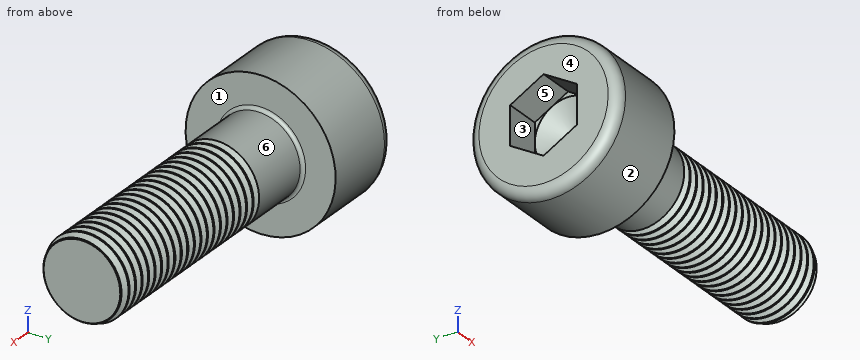
from build123d import *

# Parameters (mm, degrees)
SKETCH1_R           = 2.25
BASEHEAD_DEPTH      = 2.5
SKETCH2_R           = 1.25
BASEBODY_DEPTH      = 8
HEXAGONSOCKET_DEPTH = 1.1
HEADFILLET_R        = 0.1
TOPFILLET_R         = 0.3125
CHAMFER1_SIZE       = 0.1
LPATTERN10_COUNT    = 21
LPATTERN10_PITCH    = 0.2922


with BuildPart() as part:
    # Sketch1 → BaseHead (new body)
    with BuildSketch(Plane(origin=(0, 0, 0), x_dir=(0, 0, -1), z_dir=(1, 0, 0))):
        Circle(SKETCH1_R)
    extrude(amount=BASEHEAD_DEPTH)

    # Sketch2 → BaseBody (add)
    with BuildSketch(Plane(origin=(2.5, 0, 0), x_dir=(0, 0, -1), z_dir=(1, 0, 0))):
        Circle(SKETCH2_R)
    extrude(amount=BASEBODY_DEPTH)

    # Sketch3 → HexagonSocket (cut)
    with BuildSketch(Plane(origin=(0, 0, 0), x_dir=(0, 0, -1), z_dir=(1, 0, 0))):
        Polygon((1.154700538, 0), (0.577350269, 1), (-0.577350269, 1), (-1.154700538, 0), (-0.577350269, -1), (0.577350269, -1), align=None)
    extrude(amount=HEXAGONSOCKET_DEPTH, mode=Mode.SUBTRACT)

    # Sketch4 → Cut-Revolve1 (revolve, cut)
    with BuildSketch(Plane(origin=(-4.19613823, 0.75, 0), x_dir=(-1, 0, 0), z_dir=(0, 0, 1)), mode=Mode.PRIVATE) as cut_revolve1_sk:
        Polygon((-5.29613823, 1.75), (-5.873488499, 0.75), (-5.29613823, 0.75), align=None)
    revolve(cut_revolve1_sk.sketch.rotate(Axis((0.838992387, 0, 0), (-1, 0, 0)), 90), axis=Axis((0.838992387, 0, 0), (-1, 0, 0)), mode=Mode.SUBTRACT)

    # HeadFillet
    headfillet_edges = [part.edges().sort_by_distance(p)[0] for p in [
        (2.5, 0, 1.25),
    ]]
    fillet(headfillet_edges, radius=HEADFILLET_R)

    # TopFillet
    topfillet_edges = [part.edges().sort_by_distance(p)[0] for p in [
        (0, 0, 2.25),
    ]]
    fillet(topfillet_edges, radius=TOPFILLET_R)

    # Chamfer1
    chamfer1_edges = [part.edges().sort_by_distance(p)[0] for p in [
        (10.5, 0, 1.25),
    ]]
    chamfer(chamfer1_edges, length=CHAMFER1_SIZE)

    # Sketch5 → Cut-Revolve10 (revolve, cut)
    with BuildSketch(Plane.XY, mode=Mode.PRIVATE) as cut_revolve10_sk:
        Polygon((10.4, 1.039122814), (10.52175, 1.25), (10.52175, 1.4935), (10.27825, 1.4935), (10.27825, 1.25), align=None)
    cut_revolve10 = revolve(cut_revolve10_sk.sketch.rotate(Axis((0, 0, 0), (1, 0, 0)), 90), axis=Axis((0, 0, 0), (1, 0, 0)), mode=Mode.SUBTRACT)

    # LPattern10: Cut-Revolve10 ×21
    with Locations(*[(-i * LPATTERN10_PITCH, 0, 0) for i in range(1, LPATTERN10_COUNT)]):
        add(cut_revolve10, mode=Mode.SUBTRACT)


solid = part.part
Could you check a few things on this model? Use its own coordinates, in mm. Face numbers are marked on the shaded views. A direction names the side the tool comes from. Coordinates: 2 decimals unless noted, no trailing zeros. One line per question, with ' | ' between items.
Q1. I'm going to push a flat-ended pin straight in: P1, Ø1, axis at y = 0, z = -1.5, coming from the -X side. Where does the tip first touch, or does it pass through?
Return value:
P1: x = 0
Q2. If I drill on L1, parallel to Y at x = 0.75, z = 0.1; L2, parallel to X at y = 1.55, z = 0.15; L3, parallel to Y at x = 0.5, z = 0.85, over which ranges is the centre line in solid material (lowest first)?
Return value:
L1: -2.25 to -1, 1 to 2.25 | L2: 0 to 2.5 | L3: -2.08 to -0.53, 0.53 to 2.08
Q3. On a 3-axis mill with a long thin cutter (end or side, diameter ignored), from which of +Z, -Z, +X, -X, +Y, -Y can I reach the whole of each face in a straight line? I mean the marked faces 4, 5 and 6. Say none if no direction works.
Return value:
face 4: +Z, -Z, -X, +Y, -Y | face 5: -X | face 6: +X
Q4. Thinking about a two-plate mould opening in Z: for the marked faces 1, 2 and 3, which applies, pulls with the +Z half, pulls with the -Z half, needs draft (parallel to the pull), parting line crosses it, or undercut?
Return value:
face 1: needs draft | face 2: parting line crosses it | face 3: undercut
